from build123d import *

# Parameters (mm, degrees)
OTHER_10076_5_DEPTH = 0.5
CUT_EXTRUDE1_REACH  = 18.147


# Read off the part's stored shape, not the designer's step: 10076-5
with BuildPart() as part:
    # Other 10076-5 outline → Other 10076-5 (new body)
    with BuildSketch(Plane.XY):
        with BuildLine():
            ThreePointArc((7.573674013, -9.436602245), (7.668819519, -9.359444812), (7.763179028, -9.281328104))
            Line((7.763179028, -9.281328104), (7.919995926, -7.488902759))
            ThreePointArc((7.919995926, -7.488902759), (8.548470738, -6.76266575), (9.110578105, -5.983925684))
            ThreePointArc((9.110578105, -5.983925684), (9.242448569, -5.182849851), (8.736493865, -4.547930843))
            Line((8.736493865, -4.547930843), (8.260223146, -4.3))
            Line((8.260223146, -4.3), (5.774945887, -4.3))
            ThreePointArc((5.774945887, -4.3), (5.659072475, -4.451392897), (5.53923133, -4.5996648))
            Line((5.53923133, -4.5996648), (6.59, -6.419649523))
            ThreePointArc((6.59, -6.419649523), (5.831509763, -7.1157216), (5, -7.722693831))
            Line((5, -7.722693831), (5, -7.841555968))
            ThreePointArc((5, -7.841555968), (0, -9.3), (-5, -7.841555968))
            Line((-5, -7.841555968), (-5, -7.722693831))
            ThreePointArc((-5, -7.722693831), (-5.831509763, -7.1157216), (-6.59, -6.419649523))
            Line((-6.59, -6.419649523), (-5.53923133, -4.5996648))
            ThreePointArc((-5.53923133, -4.5996648), (-5.659072475, -4.451392897), (-5.774945887, -4.3))
            Line((-5.774945887, -4.3), (-8.260223146, -4.3))
            Line((-8.260223146, -4.3), (-10.732831081, -5.58715822))
            ThreePointArc((-10.732831081, -5.58715822), (-10.675718173, -5.6955282), (-10.617511084, -5.803314431))
            Line((-10.617511084, -5.803314431), (-9.055174855, -6.258693914))
            ThreePointArc((-9.055174855, -6.258693914), (-8.704696722, -6.64117368), (-8.882127626, -7.128661083))
            Line((-8.882127626, -7.128661083), (-9.436602245, -7.573674013))
            ThreePointArc((-9.436602245, -7.573674013), (-9.359444812, -7.668819519), (-9.281328104, -7.763179028))
            Line((-9.281328104, -7.763179028), (-7.660171598, -7.905011844))
            ThreePointArc((-7.660171598, -7.905011844), (-7.241809703, -8.211767477), (-7.320727248, -8.724502998))
            Line((-7.320727248, -8.724502998), (-7.777730077, -9.269137762))
            ThreePointArc((-7.777730077, -9.269137762), (-7.683493234, -9.347402405), (-7.588468891, -9.424709008))
            Line((-7.588468891, -9.424709008), (-5.970792243, -9.247544602))
            ThreePointArc((-5.970792243, -9.247544602), (-5.500623999, -9.466787654), (-5.477995427, -9.985067155))
            Line((-5.477995427, -9.985067155), (-5.819964104, -10.608393744))
            ThreePointArc((-5.819964104, -10.608393744), (-5.712269322, -10.666769858), (-5.603989074, -10.724052707))
            Line((-5.603989074, -10.724052707), (-4.05195869, -10.234699407))
            ThreePointArc((-4.05195869, -10.234699407), (-3.548052399, -10.358004491), (-3.424747314, -10.861910782))
            Line((-3.424747314, -10.861910782), (-3.638540174, -11.539975104))
            ThreePointArc((-3.638540174, -11.539975104), (-3.521526102, -11.576219327), (-3.404151099, -11.611277074))
            Line((-3.404151099, -11.611277074), (-1.977410637, -10.828540453))
            ThreePointArc((-1.977410637, -10.828540453), (-1.459131136, -10.851169025), (-1.239888083, -11.321337268))
            Line((-1.239888083, -11.321337268), (-1.317289186, -12.028081692))
            ThreePointArc((-1.317289186, -12.028081692), (-1.195452609, -12.04080118), (-1.073493507, -12.052286575))
            Line((-1.073493507, -12.052286575), (0.173128198, -11.006246762))
            ThreePointArc((0.173128198, -11.006246762), (0.685863719, -10.927329218), (0.992619352, -11.345691113))
            Line((0.992619352, -11.345691113), (1.054584487, -12.053955847))
            ThreePointArc((1.054584487, -12.053955847), (1.176561457, -12.042661796), (1.298417839, -12.030133462))
            Line((1.298417839, -12.030133462), (2.317013814, -10.760989181))
            ThreePointArc((2.317013814, -10.760989181), (2.804501216, -10.583558277), (3.186980982, -10.93403641))
            Line((3.186980982, -10.93403641), (3.38593107, -11.616603238))
            ThreePointArc((3.38593107, -11.616603238), (3.503360927, -11.581729673), (3.620431715, -11.545669067))
            Line((3.620431715, -11.545669067), (4.371857887, -10.10219282))
            ThreePointArc((4.371857887, -10.10219282), (4.815363304, -9.833067127), (5.258868721, -10.10219282))
            Line((5.258868721, -10.10219282), (5.58715822, -10.732831081))
            ThreePointArc((5.58715822, -10.732831081), (5.6955282, -10.675718173), (5.803314431, -10.617511084))
            Line((5.803314431, -10.617511084), (6.258693914, -9.055174855))
            ThreePointArc((6.258693914, -9.055174855), (6.64117368, -8.704696722), (7.128661083, -8.882127626))
            Line((7.128661083, -8.882127626), (7.573674013, -9.436602245))
        make_face()
    extrude(amount=OTHER_10076_5_DEPTH)

    # Sketch1 → Cut-Extrude1 (cut, up to next)
    with BuildSketch(Plane.XY.offset(0.5), mode=Mode.PRIVATE) as cut_extrude1_sk1:
        with BuildLine():
            Line((7.573674013, -9.436602245), (7.128661083, -8.882127626))
            ThreePointArc((7.128661083, -8.882127626), (6.804041546, -8.699374782), (6.443160998, -8.791795969))
            ThreePointArc((6.443160998, -8.791795969), (7.211064546, -8.173771964), (7.919995926, -7.488902759))
            Line((7.919995926, -7.488902759), (7.763179028, -9.281328104))
            ThreePointArc((7.763179028, -9.281328104), (7.668819519, -9.359444812), (7.573674013, -9.436602245))
        make_face()
    cut_extrude1_tool1 = extrude(cut_extrude1_sk1.sketch, amount=-CUT_EXTRUDE1_REACH, mode=Mode.PRIVATE) & part.part
    add(cut_extrude1_tool1.solids().sort_by_distance((7.456757, -8.533041, 0.5))[0], mode=Mode.SUBTRACT)


solid = part.part
The model under review builds one solid part; all positions refer to its coordinate system, in mm. A direction names the side the tool comes from. Coordinates: 2 decimals unless noted, no trailing zeros. Loops run counter-clockwise (first coordinate to the right, second up) from the corner with the lowest first, then second, coordinate; pieces in that order, holes last. Notation, with made-up numbers: (68, 37) -> (118, 37) arc R25 ccw to (118, 64) -> close; hole circle Ø1 at (35, -29). An arc over 180 degrees is marked (long way). Use a Markdown table: item, result. Add a question column.
1. Add section C-C on x = 1.75. Write out the cut boundary in (y, z), plus the area to 3 significant figures.
2. Add section B-B on x = 6. Write out the cut boundary in (y, z).
3. Machinability: for faces 1 (the face through (-1, -10, 0)), 2 (the face through (1.801, -11.404, 0.246)), 3 (the face through (6.06, -5.5, 0.25)), which of the approach directions +Z, -Z, +X, -X, +Y, -Y give a long, thin tool a straight path to every point of the face, cutting with its end or side? Answer none if there is none.
4. Add section A-A on y = -8.5. Write out the cut boundary in (x, z), plus the area to 3 significant figures.
5. Draft analysis for pull direction Y (two halves, no side actions). For faces 4 (the face through (-1, -10, 0.5)), 5 (the face through (-6.07, -5.52, 0.25)), 6 (the face through (-5.82, -7.125, 0.246)), 7 (the face through (-0.46, -11.54, 0.25)), state which applies: pulls with the +Y half, pulls with the -Y half, needs draft (parallel to the pull), parting line crosses it, or undercut.
6. To check wall thickness, follow line 1 (Y direction, x = -9, z = 0.25); line 2 (Y direction, x = -7.5, z = 0.45); line 3 (X direction, y = -7.25, z = 0.35). State the ranges of each line that lie inside material, in increasing order.
7. Add section D-D on x = -8. Write out the cut boundary in (y, z), plus the area to 3 significant figures.
Returned:
| question | item | result |
|---|---|---|
| 1 | outline | (-11.47, 0) -> (-9.13, 0) -> (-9.13, 0.5) -> (-11.47, 0.5) -> close |
| 1 | area | 1.17 mm² |
| 2 | outline | (-9.94, 0) -> (-6.97, 0) -> (-6.97, 0.5) -> (-9.94, 0.5) -> close; (-5.4, 0) -> (-4.3, 0) -> (-4.3, 0.5) -> (-5.4, 0.5) -> close |
| 3 | face 1 | -Z, +X, -X, +Y, -Y |
| 3 | face 2 | +Z, -Z, -Y |
| 3 | face 3 | +Z, -Z |
| 4 | outline | (-7.21, 0) -> (-3.77, 0) -> (-3.77, 0.5) -> (-7.21, 0.5) -> close; (3.77, 0) -> (6.82, 0) -> (6.82, 0.5) -> (3.77, 0.5) -> close |
| 4 | area | 3.24 mm² |
| 5 | face 4 | needs draft |
| 5 | face 5 | undercut |
| 5 | face 6 | undercut |
| 5 | face 7 | pulls with the -Y half |
| 6 | line 1 | y = -7.79 to -7.22, -6.28 to -4.69 |
| 6 | line 2 | y = -9.42 to -8.94, -7.95 to -4.3 |
| 6 | line 3 | x = -9.03 to -5.66, 5.66 to 8.14 |
| 7 | outline | (-7.88, 0) -> (-4.3, 0) -> (-4.3, 0.5) -> (-7.88, 0.5) -> close |
| 7 | area | 1.79 mm² |
